Check sheet for the modelled part. Datum: model origin and axes. Units: mm. Round coordinates to 2 decimals unless told otherwise and drop trailing zeros. Loops run counter-clockwise (first coordinate to the right, second up) from the corner with the lowest first, then second, coordinate; pieces in that order, holes last. Notation, with made-up numbers: (15.5, 53) - (74.5, 53) arc R16 ccw to (74.5, 74) - close; hole circle Ø4 at (45.5, 15). An arc over 180 degrees is marked (long way). Put each result on its own line as item: value. Start each with the question number.
Item 1: Material ranges on line 1 along X through (y, z) = (1.35, -73.5); line 2 along Z through (x, y) = (-70, 2.2); line 3 along X through (y, z) = (0.25, 5), recorded low to high.
Item 2: Section check B-B, the plane z = 78.5. Record the cut outline in (x, y), and give its area (3 significant figures).
Item 3: Section check A-A, the plane y = 0.6. Record the cut outline in (x, z), and give its area (3 significant figures).
Item 4: Gauge pin test, flat ends, axial feed: pin 1 Ø2 at (y, z) = (1, 161) entering from -X; pin 2 Ø1.5 at (y, z) = (2.5, -3) entering from -X. Record the tip position at first contact, or that the pin passes through.
Item 5: Draft check along X on faces 1 (the conical face through (-76.989, 2.125, 176.748)), 2 (the flat face through (-38, 4, 54)), 3 (the conical face through (-28.989, 2.125, 176.748)). Enter one of: pulls with the +X half, pulls with the -X half, needs draft (parallel to the pull), parting line crosses it, or undercut.
Autodesk Inventor part; units mm, degrees
ref_plane "YZ Plane" through (0, 0, 0) normal (1, 0, 0) x (0, 1, 0)
ref_plane "XZ Plane" through (0, 0, 0) normal (0, 1, 0) x (-1, 0, 0)
ref_plane "XY Plane" through (0, 0, 0) normal (0, 0, 1) x (1, 0, 0)
sketch "Эскиз1" plane through (0, 0, 0) normal (0, 1, 0) x (-1, 0, 0)
  line L0 (-2.6795, -79) -> (80.3545, -79)
  line L1 (-2.6795, 184) -> (80.3545, 184)
  circle A0 centre (28.0773, 178.5) radius 1.85
  circle A1 centre (76.0773, 178.5) radius 1.85
  circle A2 centre (76.0773, -73.5) radius 1.85
  circle A3 centre (28.0773, -73.5) radius 1.85
  line L2 (80.3545, 184) -> (-2.6795, 184)
  line L3 (-2.6795, 184) -> (-2.6795, -79)
  line L4 (-2.6795, -79) -> (80.3545, -79)
  line L5 (80.3545, -79) -> (80.3545, 184)
  point P0 (0, 0)
  point P1 (83.0251, -19)
  dimension "d7" = 5.5
  dimension "d8" = 48
  dimension "d9" = 4.2772
  dimension "d10" = 5.5
  dimension "d11" = 263
  dimension "d12" = 83.034
extrude "Выдавливание1" add sketch "Эскиз1" along normal blind 4
chamfer "Фаска1" distance 2 angle 45 4 edges at (-74.2273, 4, 178.5) (-26.2273, 4, 178.5) (-26.2273, 4, -73.5) (-74.2273, 4, -73.5)
sketch "Эскиз2" plane through (0, 4, 0) normal (0, 1, 0) x (1, 0, 0)
  line L0 (-74.9909, -157.5) -> (-74.9909, 52.5)
  line L1 (-74.9909, 52.5) -> (-54.9909, 52.5)
  line L2 (-54.9909, -157.5) -> (-74.9909, -157.5)
  line L3 (-54.9909, 57.5) -> (-74.9909, 57.5)
  line L4 (-74.9909, 57.5) -> (-79.9909, 57.5)
  line L5 (-79.9909, 57.5) -> (-79.9909, -162.5)
  line L6 (-79.9909, -162.5) -> (-74.9909, -162.5)
  line L7 (-74.9909, -162.5) -> (-54.9909, -162.5)
  line L8 (-54.9909, -162.5) -> (-54.9909, -157.5)
  line L9 (-54.9909, 52.5) -> (-54.9909, 57.5)
  point P0 (0, 0)
extrude "Выдавливание2" cut sketch "Эскиз2" against normal blind 10
thicken "Толщина2" operation add thickness 1 both sides no extend neighbours yes toward (-1, 0, 0) faces at (-79.9909, 2.6667, 15.8333)
properties part number "KB33-046-004-002 - Передняя пластина" material "Дерево (вишня)"
Check result:
1. line 1: -80.35 to -77.93, -74.23 to -29.93, -26.23 to 2.68
1. line 2: -79 to -57.5, -52.5 to 157.5, 162.5 to 184
1. line 3: -74.99 to 2.68
2. outline: (-74.99, 0) - (2.68, 0) - (2.68, 4) - (-74.99, 4) - close
2. area: 311 mm²
3. outline: (-80.35, -79) - (2.68, -79) - (2.68, 184) - (-80.35, 184) - (-80.35, 162.5) - (-54.99, 162.5) - (-54.99, 157.5) - (-74.99, 157.5) - (-74.99, -52.5) - (-54.99, -52.5) - (-54.99, -57.5) - (-80.35, -57.5) - close; hole circle Ø3.7 at (-76.08, -73.5); hole circle Ø3.7 at (-76.08, 178.5); hole circle Ø3.7 at (-28.08, -73.5); hole circle Ø3.7 at (-28.08, 178.5)
3. area: 20,400 mm²
4. pin 1: x = -54.99
4. pin 2: x = -74.99
5. face 1: undercut
5. face 2: needs draft
5. face 3: undercut
